For this review, use the dimensioned drawing (mm, ordinates from the lowest corner) and the shaded views. A direction names the side the tool comes from. Coordinates: 2 decimals unless noted, no trailing zeros. Order: outer loops, then holes, each group sorted by start corner. A loop starts at its lowest first (then second) coordinate and runs counter-clockwise, first axis right, second up. Notation, with made-up numbers: M -5.5,6 L 51.5,6 A19 ccw 51.5,23 Z; hole C 72.5,7 d10. An arc over 180 degrees is marked long. Answer as CSV lines item,"result". Start each with the question number.
Q1. Consider section C-C on z = 2.5. Write out the cut boundary in (x, y), and give its area (3 significant figures).
Q2. The part is to be moulded in two halves that separate along Y. For the marked faces 1, 2 and 3, say which applies: +Y half, -Y half, draft (parallel to the pull), parting line (faces both ways), or undercut.
Q3. Machinability: for the marked faces 4 and 5, which of the approach directions +Z, -Z, +X, -X, +Y, -Y give a long, thin tool a straight path to every point of the face, cutting with its end or side? Answer none if there is none.
Q4. For P1, Ø4, axis at x = 6.5, y = 6, coming from the +Z side; P2, Ø1.5, axis at y = 3, z = 5, coming from the -X side; P3, Ø2.5, axis at x = 5, y = 5, coming from the -Z side, all flat-tipped, find the tip position at first contact; note any pin that passes through.
Q5. Consider section D-D on x = 1.25. Write out the cut boundary in (y, z).
Q6. Wall thickness on L1, parallel to Y at x = 5, z = 1.8; L2, parallel to Y at x = 5, z = 7.45; L3, parallel to X at y = 4.75, z = 1.75: over which ranges is each line inside the solid? List them lowest first. Write a range as [from, to].
Q7. Consider section A-A on y = 5. Write out the cut boundary in (x, z).
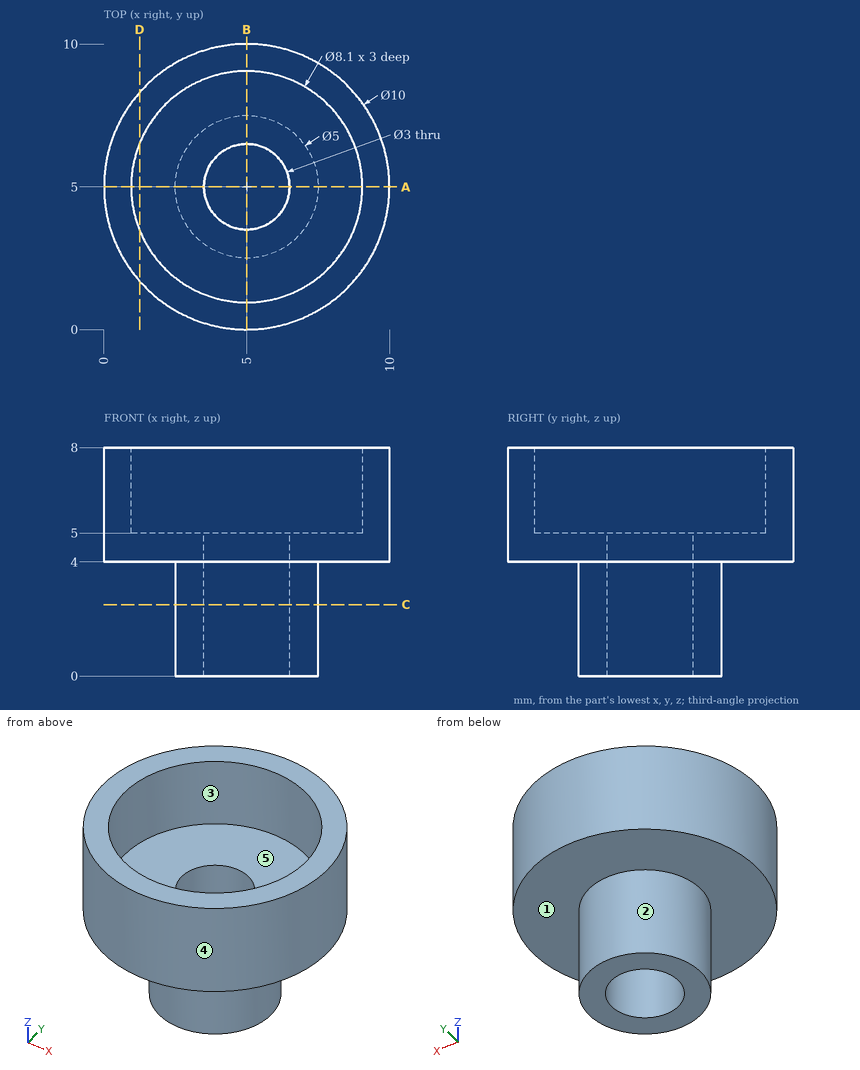
Evaluation:
1,outline,"C 5,5 d5; hole C 5,5 d3"
1,area,"12.6 mm²"
2,face 1,"draft"
2,face 2,"parting line"
2,face 3,"undercut"
3,face 4,"+Z, -Z"
3,face 5,"+Z"
4,P1,"stops at z = 5"
4,P2,"stops at x = 0.16"
4,P3,"passes through"
5,outline,"M 1.69,4 L 8.31,4 L 8.31,8 L 6.53,8 L 6.53,5 L 3.47,5 L 3.47,8 L 1.69,8 Z"
6,L1,"y = [2.5, 3.5], [6.5, 7.5]"
6,L2,"y = [0, 0.95], [9.05, 10]"
6,L3,"x = [2.51, 3.52], [6.48, 7.49]"
7,outline,"M 0,4 L 2.5,4 L 2.5,0 L 3.5,0 L 3.5,5 L 0.95,5 L 0.95,8 L 0,8 Z; M 6.5,0 L 7.5,0 L 7.5,4 L 10,4 L 10,8 L 9.05,8 L 9.05,5 L 6.5,5 Z"
